Source: three-view drawing plus pictorial views. Frame: mm from the lowest corner of the part. A direction names the side the tool comes from. Give positions to 0.01 mm unless a question says otherwise; leave off trailing zeros. Loops run counter-clockwise (first coordinate to the right, second up) from the corner with the lowest first, then second, coordinate; pieces in that order, holes last. Notation, with made-up numbers: M 41,-21 L 88,-21 A29 ccw 88,3 Z; hole C 71,71.5 d8. An arc over 180 degrees is marked long. One line per item, written item: value. Start each with the question number.
(1) Pull-direction query (Y, two-part tool) for the marked faces 4, 5, 6 and 7; classes: released by +Y, released by -Y, zero draft, split by the parting line, or undercut.
(2) Section B-B on x = 48.5. Output: boundary loops of the cut face in (y, z).
(3) Ray query, line 1 along X through (y, z) = (41.5, 0.5); line 2 along X through (y, z) = (27.5, 3.25) (1 decimal); line 3 along Y through (x, z) = (59, 2.5). Return the intervals inside material, ascending. Write a range as from..to.
(4) Section A-A on z = 4. Output: boundary loops of the cut face in (x, y), plus the area to 3 significant figures.
(5) Section D-D on x = 58. Output: boundary loops of the cut face in (y, z), plus the area to 3 significant figures.
(6) Pin query (flat end, axial travel): P1, Ø2, axis at x = 65, y = 31, coming from the -Z side; P2, Ø1.5, axis at x = 43.5, z = 1, coming from the +Y side; P3, Ø3, axis at x = 24, z = 2, coming from the -Y side. Return the tip coordinate at first contact, or that it passes through.
(7) Access query for the marked faces 1, 2 and 3. Directions: +Z, -Z, +X, -X, +Y, -Y. A direction counts if a zero-diameter tool reaches every point of the face in a straight line with its end or side. Return the directions, or none.
(8) Section C-C on y = 47. Output: boundary loops of the cut face in (x, z), plus the area to 3 significant figures.
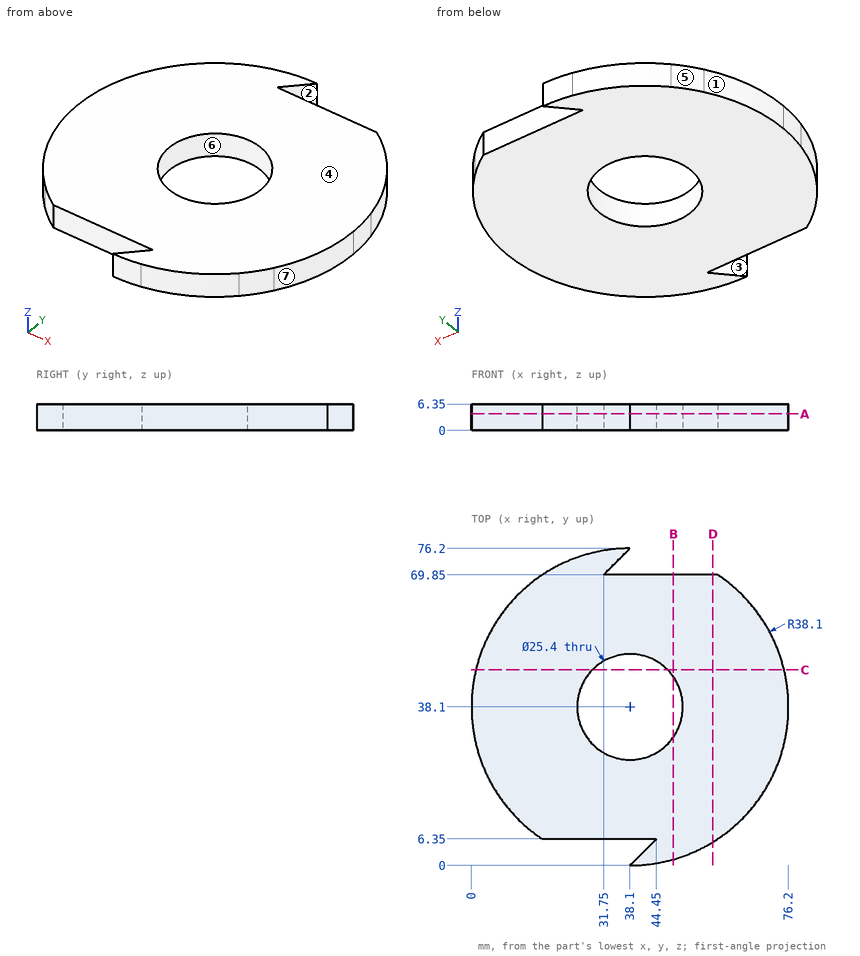
Output values:
1. face 4: zero draft
1. face 5: released by +Y
1. face 6: undercut
1. face 7: released by -Y
2. outline: M 1.45,0 L 30.81,0 L 30.81,6.35 L 1.45,6.35 Z; M 45.39,0 L 69.85,0 L 69.85,6.35 L 45.39,6.35 Z
3. line 1: x = 0.15..25.86, 50.34..76.05
3. line 2: x = 1.5..31.1, 45.1..74.7
3. line 3: y = 6.24..69.85
4. outline: M 0,38.1 A38.1 ccw 0.76,30.54 A38.1 ccw 11.16,11.16 A38.1 ccw 17.04,6.35 L 44.45,6.35 L 38.1,0 A38.1 ccw 45.26,0.68 A38.1 ccw 64.75,10.87 A38.1 ccw 69.85,17.04 A38.1 ccw 76.2,38.1 A38.1 ccw 75.44,45.66 A38.1 ccw 65.04,65.04 A38.1 ccw 59.16,69.85 L 31.75,69.85 L 38.1,76.2 A38.1 ccw 30.54,75.44 A38.1 ccw 11.16,65.04 A38.1 ccw 6.35,59.16 A38.1 ccw Z; hole C 38.1,38.1 d25.4
4. area: 3,830 mm²
5. outline: M 5.61,0 L 69.85,0 L 69.85,6.35 L 5.61,6.35 Z
5. area: 408 mm²
6. P1: stops at z = 0
6. P2: stops at y = 69.85
6. P3: stops at y = 6.35
7. face 1: +Z, -Z, -X, +Y
7. face 2: +Z, -Z, +X
7. face 3: +Z, -Z, -X
8. outline: M 1.05,0 L 29.04,0 L 29.04,6.35 L 1.05,6.35 Z; M 47.16,0 L 75.15,0 L 75.15,6.35 L 47.16,6.35 Z
8. area: 355 mm²
